Work out the finished part from the listing and answer in its coordinate system (mm). Round coordinates to 2 decimals unless told otherwise and drop trailing zeros. Order: outer loops, then holes, each group sorted by start corner. A loop starts at its lowest first (then second) coordinate and runs counter-clockwise, first axis right, second up. Notation, with made-up numbers: (2, 78) - (52, 78) arc R18 ccw to (52, 91) - close; hole circle Ø7 at (-32.75, 9.5). An arc over 180 degrees is marked (long way). Put each result on its own line as item: value.
```python
from build123d import *

# Parameters (mm, degrees)
F2_SIZE = 0.5


with BuildPart() as f1:
    # F0 (on Right) → F1 (revolve)
    with BuildSketch(Plane.YZ):
        with BuildLine():
            Line((-5.125, 0), (0, 0))
            Line((0, 0), (0, 1.125))
            ThreePointArc((0, 1.125), (-0.088388, 1.161612), (-0.125, 1.25))
            Line((-0.125, 1.25), (-5.125, 1.25))
            Line((-5.125, 1.25), (-5.125, 0))
        make_face()
        with BuildLine():
            Line((0, 1.125), (0, 0))
            Line((0, 0), (5.125, 0))
            Line((5.125, 0), (5.125, 1.25))
            Line((5.125, 1.25), (0.125, 1.25))
            ThreePointArc((0.125, 1.25), (0.088388, 1.161612), (0, 1.125))
        make_face()
    revolve(axis=Axis((0, 2.5625, 0), (0, -1, 0)))

    # F2
    f2_edges = [f1.edges().sort_by_distance(p)[0] for p in [
        (0, -5.125, -1.25),
        (0, 5.125, -1.25),
    ]]
    chamfer(f2_edges, length=F2_SIZE)


solid = f1.part
```
1) A cutting plane is placed at A-A on x = 0. Write down the section's boundary in (y, z) (3 decimals).
Findings below:
outline: (-5.125, -0.75) - (-4.625, -1.25) - (-0.125, -1.25) arc R0.125 cw to (0, -1.125) arc R0.125 cw to (0.125, -1.25) - (4.625, -1.25) - (5.125, -0.75) - (5.125, 0.75) - (4.625, 1.25) - (0.125, 1.25) arc R0.125 cw to (0, 1.125) arc R0.125 cw to (-0.125, 1.25) - (-4.625, 1.25) - (-5.125, 0.75) - close
2) A cutting plane is placed at C-C on y = 1. Write down the section's boundary in (x, z).
Findings below:
outline: circle Ø2.5 at (0, 0)
3) A cutting plane is placed at B-B on z = 0. Write down the section's boundary in (x, y) (3 decimals).
Findings below:
outline: (-1.25, -4.625) - (-0.75, -5.125) - (0.75, -5.125) - (1.25, -4.625) - (1.25, -0.125) arc R0.125 cw to (1.125, 0) arc R0.125 cw to (1.25, 0.125) - (1.25, 4.625) - (0.75, 5.125) - (-0.75, 5.125) - (-1.25, 4.625) - (-1.25, 0.125) arc R0.125 cw to (-1.125, 0) arc R0.125 cw to (-1.25, -0.125) - close
4) Straight lines are drawn through the part: L1, parallel to Y at x = -0.8, z = -0.9; L2, parallel to X at y = -4.5, z = -0.3; L3, parallel to X at y = -3.5, z = -1. For each, find the intervals that lie inside material, in ascending order. Write a range as from..to.
Findings below:
L1: y = -4.67..-0.12, 0.12..4.67
L2: x = -1.21..1.21
L3: x = -0.75..0.75
